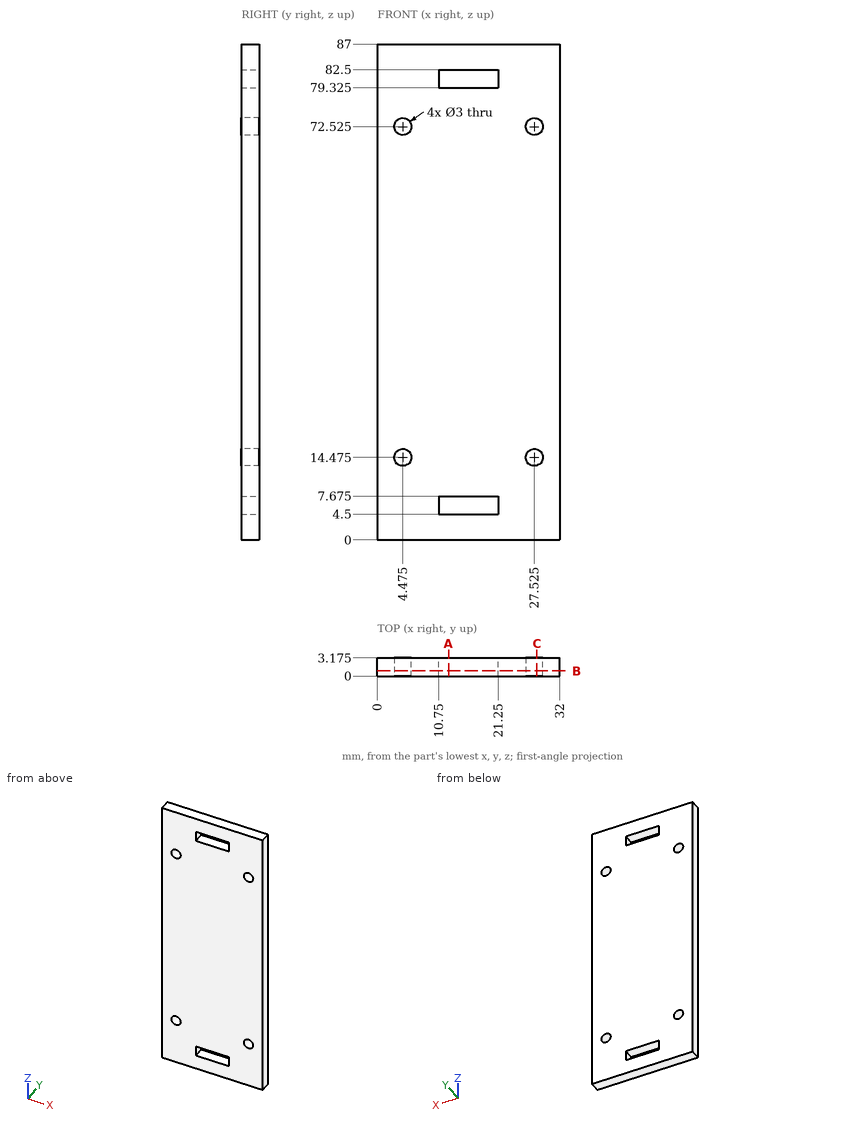
Answer from the drawing. Dimensions are ordinates in mm from the lowest x, y and z of the part. Coordinates: 2 decimals unless noted, no trailing zeros. Order: outer loops, then holes, each group sorted by start corner. A loop starts at its lowest first (then second) coordinate and runs counter-clockwise, first axis right, second up. Notation, with made-up numbers: (-35, 78) - (5, 78) arc R24 ccw to (5, 114) - close; hole circle Ø11 at (50, -20). An arc over 180 degrees is marked (long way). Put each result on its own line as item: value. Start each with the question number.
1) Find the intervals of material crossed by line 1 (Z direction, x = 20, y = 2.9) (3 decimals); line 2 (X direction, y = 0.35, z = 71.5); line 3 (Z direction, x = 5, y = 2.3), in increasing order. Write a range as from..to.
2) Find section B-B (y = 0.9). Give the vertices of the cut face in (x, z) (3 decimals), plus the area to 3 significant figures.
3) A flat-ended cylindrical pin translates along its axis: pin 1 (4 mm diameter, centred on x = 27.525, z = 14.475, fed in from +Y) (3 decimals). Find the tip coordinate at first contact, or state that the pin passes through.
4) Find section C-C (x = 28). Give the vertices of the cut face in (y, z) (3 decimals), plus the area to 3 significant figures.
5) Find section A-A (x = 12.5). Give the vertices of the cut face in (y, z) (3 decimals).
Results list:
1. line 1: z = 0..4.5, 7.675..79.325, 82.5..87
1. line 2: x = 0..3.38, 5.57..26.43, 28.62..32
1. line 3: z = 0..13.07, 15.88..71.12, 73.93..87
2. outline: (0, 0) - (32, 0) - (32, 87) - (0, 87) - close; hole circle Ø3 at (4.475, 14.475); hole circle Ø3 at (4.475, 72.525); hole (10.75, 4.5) - (21.25, 4.5) - (21.25, 7.675) - (10.75, 7.675) - close; hole (10.75, 79.325) - (21.25, 79.325) - (21.25, 82.5) - (10.75, 82.5) - close; hole circle Ø3 at (27.525, 14.475); hole circle Ø3 at (27.525, 72.525)
2. area: 2,690 mm^2
3. pin 1: stops at y = 3.175
4. outline: (0, 0) - (3.175, 0) - (3.175, 13.052) - (0, 13.052) - close; (0, 15.898) - (3.175, 15.898) - (3.175, 71.102) - (0, 71.102) - close; (0, 73.948) - (3.175, 73.948) - (3.175, 87) - (0, 87) - close
4. area: 258 mm^2
5. outline: (0, 0) - (3.175, 0) - (3.175, 4.5) - (0, 4.5) - close; (0, 7.675) - (3.175, 7.675) - (3.175, 79.325) - (0, 79.325) - close; (0, 82.5) - (3.175, 82.5) - (3.175, 87) - (0, 87) - close
